Could you check a few things on this model? Use its own coordinates, in mm. A direction names the side the tool comes from. Coordinates: 2 decimals unless noted, no trailing zeros. Loops run counter-clockwise (first coordinate to the right, second up) from the corner with the lowest first, then second, coordinate; pieces in that order, holes last. Notation, with made-up numbers: (-3.5, 64) -> (55.5, 64) arc R22 ccw to (55.5, 90) -> close; hole circle Ø3 at (62.5, 4). An arc over 180 degrees is marked (long way). One line per question, with ' | ' between items. Start each with the question number.
(1) If I drill on line 1 along X through (y, z) = (17.25, 9); line 2 along Z through (x, y) = (-3, 14.75), over which ranges is the centre line in solid material (lowest first)?
(2) Suppose I cut it at A-A (y = 15.5). Please give me the cut outline in (x, z), plus the area to 3 significant figures.
(3) I'm going to push flat-ended pins straight in: pin 1 Ø3 at (x, y) = (-1, 20.5) entering from -Z; pin 2 Ø1.4 at (x, y) = (3.5, 21.5) entering from +Z; pin 3 Ø3 at (y, z) = (22, 0.5) entering from +X; pin 4 Ø3 at (x, z) = (9, -9) entering from +Y. Where does each tip first touch, or does it pass through?
(4) Suppose I cut it at B-B (x = 0). Please give me the cut outline in (y, z), plus the area to 3 significant figures.
(5) Which directions (+Z, -Z, +X, -X, +Y, -Y) give clear straight access to the entire face, cutting with the end or side of a thin tool? Please do faces 5 (the face through (6, 22.8, 4)), 6 (the face through (3.2, 13, -2.9)), 7 (the face through (0, 21, 9.046)).
(6) Suppose I cut it at C-C (x = 8). Please give me the cut outline in (y, z).
(7) Suppose I cut it at D-D (z = -7.75). Please give me the cut outline in (x, y).
(8) If we mould it in two halves opening along X, with no side actions, what happens to faces 1 (the face through (7.58, 11.56, -8.26)), 2 (the face through (-8.85, 21, 0)), 3 (the face through (8.85, 21, 0)), 4 (the face through (0, 21, -9.046))? For each: pulls with the +X half, pulls with the -X half, needs draft (parallel to the pull), parting line crosses it, or undercut.
```python
from build123d import *

# Parameters (mm, degrees)
SKETCH1_W               = 25
SKETCH1_H               = 25
BOSS_EXTRUDE1_DEPTH     = 20
SKETCH4_R               = 4.15
CUT_EXTRUDE2_DEPTH      = 21
CUT_EXTRUDE3_DEPTH      = 7
SKETCH9_W               = 17.7
SKETCH9_H               = 18.092678694
BOSS_EXTRUDE3_DEPTH     = 2.8
SKETCH6_R               = 1.6
CUT_EXTRUDE4_DEPTH      = 3.8
CUT_EXTRUDE4_DEPTH_BACK = 21


with BuildPart() as part:
    # Sketch1 → Boss-Extrude1 (new body)
    with BuildSketch(Plane(origin=(0, 0, 0), x_dir=(1, 0, 0), z_dir=(0, 1, 0))):
        Rectangle(SKETCH1_W, SKETCH1_H)
    extrude(amount=BOSS_EXTRUDE1_DEPTH)

    # Sketch4 → Cut-Extrude2 (cut, through all)
    with BuildSketch(Plane(origin=(0, 20, 0), x_dir=(1, 0, 0), z_dir=(0, 1, 0))):
        with Locations(Location((0, 0, 0), (0, 0, 270))):  # turned: the seam where the file's is
            Circle(SKETCH4_R)
    extrude(amount=-CUT_EXTRUDE2_DEPTH, mode=Mode.SUBTRACT)

    # Sketch5 → Cut-Extrude3 (cut)
    with BuildSketch(Plane(origin=(0, 20, 0), x_dir=(1, 0, 0), z_dir=(0, 1, 0))):
        Polygon((-3.7, -6.408587988), (3.7, -6.408587988), (7.4, 0), (3.7, 6.408587988), (-3.7, 6.408587988), (-7.4, 0), align=None)
    extrude(amount=-CUT_EXTRUDE3_DEPTH, mode=Mode.SUBTRACT)

    # Sketch9 → Boss-Extrude3 (add)
    with BuildSketch(Plane(origin=(0, 20, 0), x_dir=(1, 0, 0), z_dir=(0, 1, 0))):
        Rectangle(SKETCH9_W, SKETCH9_H)
        Polygon((-3.7, -6.408587988), (3.7, -6.408587988), (7.4, 0), (3.7, 6.408587988), (-3.7, 6.408587988), (-7.4, 0), align=None, mode=Mode.SUBTRACT)
    extrude(amount=BOSS_EXTRUDE3_DEPTH)

    # Sketch6 → Cut-Extrude4 (cut, two sides)
    with BuildSketch(Plane(origin=(0, 20, 0), x_dir=(1, 0, 0), z_dir=(0, 1, 0))) as cut_extrude4_sk:
        with Locations(Location((9, -9, 0), (0, 0, 270))):  # turned: the seam where the file's is
            Circle(SKETCH6_R)
        with Locations(Location((-9, -9, 0), (0, 0, 270))):  # turned: the seam where the file's is
            Circle(SKETCH6_R)
        with Locations(Location((-9, 9, 0), (0, 0, 270))):  # turned: the seam where the file's is
            Circle(SKETCH6_R)
        with Locations(Location((9, 9, 0), (0, 0, 270))):  # turned: the seam where the file's is
            Circle(SKETCH6_R)
    extrude(amount=CUT_EXTRUDE4_DEPTH, mode=Mode.SUBTRACT)
    extrude(cut_extrude4_sk.sketch, amount=-CUT_EXTRUDE4_DEPTH_BACK, mode=Mode.SUBTRACT)


solid = part.part
```
Checks:
1) line 1: x = -12.5 to -10.6, -7.4 to 7.4, 10.6 to 12.5 | line 2: z = -12.5 to -6.41, 6.41 to 12.5
2) outline: (-12.5, -12.5) -> (12.5, -12.5) -> (12.5, 12.5) -> (-12.5, 12.5) -> close; hole circle Ø3.2 at (-9, -9); hole circle Ø3.2 at (-9, 9); hole (-7.4, 0) -> (-3.7, -6.41) -> (3.7, -6.41) -> (7.4, 0) -> (3.7, 6.41) -> (-3.7, 6.41) -> close; hole circle Ø3.2 at (9, -9); hole circle Ø3.2 at (9, 9) | area: 451 mm^2
3) pin 1: stops at z = -12.5 | pin 2: stops at z = 9.05 | pin 3: stops at x = 8.85 | pin 4: passes through
4) outline: (0, -12.5) -> (20, -12.5) -> (20, -9.05) -> (22.8, -9.05) -> (22.8, -6.41) -> (13, -6.41) -> (13, -4.15) -> (0, -4.15) -> close; (0, 4.15) -> (13, 4.15) -> (13, 6.41) -> (22.8, 6.41) -> (22.8, 9.05) -> (20, 9.05) -> (20, 12.5) -> (0, 12.5) -> close | area: 317 mm^2
5) face 5: +Z, -Z, +X, -X, +Y | face 6: +Y | face 7: +Z, +X, -X, +Y
6) outline: (0, -12.5) -> (20, -12.5) -> (20, -10.25) -> (0, -10.25) -> close; (0, -7.75) -> (22.8, -7.75) -> (22.8, 7.75) -> (0, 7.75) -> close; (0, 10.25) -> (20, 10.25) -> (20, 12.5) -> (0, 12.5) -> close
7) outline: (-12.5, 0) -> (-10, 0) -> (-10, 20) -> (-12.5, 20) -> close; (-8, 0) -> (8, 0) -> (8, 22.8) -> (-8, 22.8) -> close; (10, 0) -> (12.5, 0) -> (12.5, 20) -> (10, 20) -> close
8) face 1: undercut | face 2: pulls with the -X half | face 3: pulls with the +X half | face 4: needs draft
